Answer from the drawing. Dimensions are ordinates in mm from the lowest x, y and z of the part. A direction names the side the tool comes from. Round coordinates to 2 decimals unless told otherwise and drop trailing zeros. Loops run counter-clockwise (first coordinate to the right, second up) from the corner with the lowest first, then second, coordinate; pieces in that order, holes last.
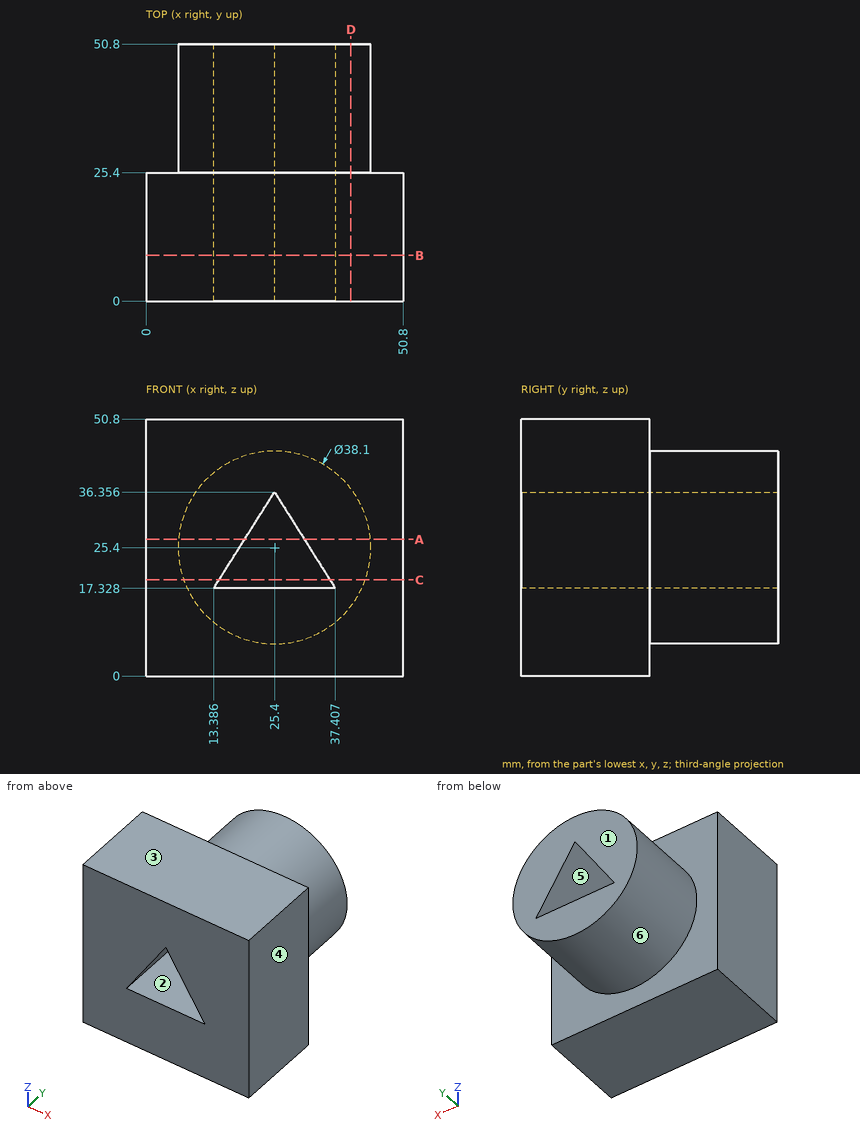
1. Consider probe 1 along Z at (x, y) = (34, 34.5) (1 decimal); probe 2 along Y at (x, z) = (10, 5); probe 3 along Z at (x, y) = (24, 47) (1 decimal). Determine where each line is inside the solid, lowest interval first.
Answer key:
probe 1: z = 8.4 to 17.3, 22.7 to 42.4
probe 2: y = 0 to 25.4
probe 3: z = 6.4 to 17.3, 34.1 to 44.4
2. Find section C-C (z = 19). Write down the section's boundary in (x, y), then the cut area to 3 significant figures.
Answer key:
outline: (0, 0) - (14.44, 0) - (14.44, 50.8) - (7.46, 50.8) - (7.46, 25.4) - (0, 25.4) - close; (36.35, 0) - (50.8, 0) - (50.8, 25.4) - (43.34, 25.4) - (43.34, 50.8) - (36.35, 50.8) - close
area: 1,090 mm2
3. Find section B-B (y = 9). Write down the section's boundary in (x, z) (1 decimal).
Answer key:
outline: (0, 0) - (50.8, 0) - (50.8, 50.8) - (0, 50.8) - close; hole (13.4, 17.3) - (37.4, 17.3) - (25.4, 36.4) - close
4. Find section D-D (x = 40.5). Write down the section's boundary in (y, z) (1 decimal).
Answer key:
outline: (0, 0) - (25.4, 0) - (25.4, 13.8) - (50.8, 13.8) - (50.8, 37) - (25.4, 37) - (25.4, 50.8) - (0, 50.8) - close
5. Determine the mould class of the marked faces 1, 2 and 3 for opening direction Z: +Z half, -Z half, draft (parallel to the pull), parting line (faces both ways), or undercut.
Answer key:
face 1: draft
face 2: undercut
face 3: +Z half
6. Which of the six approach directions +Z, -Z, +X, -X, +Y, -Y give full straight-line access (tool end or side, diameter ignored) to the marked faces 4, 5 and 6?
Answer key:
face 4: +Z, -Z, +X, +Y, -Y
face 5: +Y, -Y
face 6: +Y
7. Find section A-A (z = 27). Write down the section's boundary in (x, y).
Answer key:
outline: (0, 0) - (19.49, 0) - (19.49, 50.8) - (6.42, 50.8) - (6.42, 25.4) - (0, 25.4) - close; (31.3, 0) - (50.8, 0) - (50.8, 25.4) - (44.38, 25.4) - (44.38, 50.8) - (31.3, 50.8) - close
8. Given pin 1 (4 mm diameter, centred on y = 36.5, z = 11, fed in from +X); pin 2 (12 mm diameter, centred on x = 24.5, y = 34.5, fed in from +Z); pin 3 (1 mm diameter, centred on x = 16, y = 34.5, fed in from -Z), each flat-ended and moving along its own axis, determine where each tip first touches the part or whether it passes through.
Answer key:
pin 1: stops at x = 39.86
pin 2: stops at z = 44.45
pin 3: stops at z = 8.56
